For this review, take the finished solid that the model builds, in its own axes (mm). Face numbers are marked on the shaded views. A direction names the side the tool comes from. Coordinates: 2 decimals unless noted, no trailing zeros. Write each loop counter-clockwise with the first axis right and the second up, starting at its lowest first coordinate (ties: lowest second). Pieces come first, ordered by that corner, then holes.
```python
from build123d import *

# Parameters (mm, degrees)
SKETCH_A01_8_R     = 6.85
SKETCH_A01_8_W     = 10
SKETCH_A01_8_H     = 10
EXTRUDE1_DEPTH     = 100
CUT_EXTRUDE1_DEPTH = 101
CIRPATTERN1_COUNT  = 2
CIRPATTERN1_ANGLE  = 90
CUT_EXTRUDE2_DEPTH = 101
EXTRUDE3_DEPTH     = 100


with BuildPart() as part:
    # Sketch A01-8 → Extrude1 (new body)
    with BuildSketch(Plane.XY):
        Polygon((-16.5, -11), (-16.5, -9.5), (-15.863961, -9.5), (-10.14602885, -3.78206785), (-10.14602885, 3.78206785), (-15.863961, 9.5), (-16.5, 9.5), (-16.5, 11), (-21, 11), (-21, 4), (-25, 4), (-25, 25), (25, 25), (25, 4), (21, 4), (21, 11), (16.5, 11), (16.5, 9.5), (15.863961, 9.5), (10.14602885, 3.78206785), (10.14602885, -3.78206785), (15.863961, -9.5), (16.5, -9.5), (16.5, -11), (21, -11), (21, -4), (25, -4), (25, -25), (4, -25), (4, -21), (11, -21), (11, -16.5), (9.5, -16.5), (9.5, -15.863961), (3.78206785, -10.14602885), (-3.78206785, -10.14602885), (-9.5, -15.863961), (-9.5, -16.5), (-11, -16.5), (-11, -21), (-4, -21), (-4, -25), (-25, -25), (-25, -4), (-21, -4), (-21, -11), align=None)
        Circle(SKETCH_A01_8_R, mode=Mode.SUBTRACT)
        with Locations((-18, -18)):
            Rectangle(SKETCH_A01_8_W, SKETCH_A01_8_H, mode=Mode.SUBTRACT)
        with Locations((18, -18)):
            Rectangle(SKETCH_A01_8_W, SKETCH_A01_8_H, mode=Mode.SUBTRACT)
        Polygon((23, 13), (16.535534, 13), (14.035536811, 10.500002811), (-14.035536811, 10.500002811), (-16.535534, 13), (-23, 13), (-23, 23), (23, 23), align=None, mode=Mode.SUBTRACT)
    extrude(amount=-EXTRUDE1_DEPTH)

    # Sketch1 → Cut-Extrude1 (cut, through all)
    with BuildSketch(Plane.XY):
        Polygon((-16.5, -13), (-9.340048075, -5.840048075), (-5.840048075, -9.340048075), (-13, -16.5), align=None)
    cut_extrude1 = extrude(amount=-CUT_EXTRUDE1_DEPTH, mode=Mode.SUBTRACT)

    # CirPattern1: Cut-Extrude1 ×2 about axis
    cirpattern1_axis = Axis((0, 0, 0), (0, 0, 1))
    for i in range(1, CIRPATTERN1_COUNT):
        add(cut_extrude1.rotate(cirpattern1_axis, i * CIRPATTERN1_ANGLE / (CIRPATTERN1_COUNT - 1)), mode=Mode.SUBTRACT)

    # Sketch2 → Cut-Extrude2 (cut, through all)
    with BuildSketch(Plane.XY):
        with BuildLine():
            Line((-14.035536811, 10.500002811), (-10.114441476, 6.578907476))
            ThreePointArc((-10.114441476, 6.578907476), (0, 10.768446311), (10.114441476, 6.578907476))
            Line((10.114441476, 6.578907476), (14.035536811, 10.500002811))
            ThreePointArc((14.035536811, 10.500002811), (0, 16.313712513), (-14.035536811, 10.500002811))
        make_face()
    extrude(amount=-CUT_EXTRUDE2_DEPTH, mode=Mode.SUBTRACT)

    # Sketch3 → Extrude3 (add, through all)
    with BuildSketch(Plane.XY):
        Polygon((-11, 23), (-11, 15), (-7, 15), (-7, 17), (-9.5, 17), (-9.5, 23), align=None)
        Polygon((11, 23), (11, 15), (7, 15), (7, 17), (9.5, 17), (9.5, 23), align=None)
    extrude(amount=-EXTRUDE3_DEPTH)


solid = part.part
```
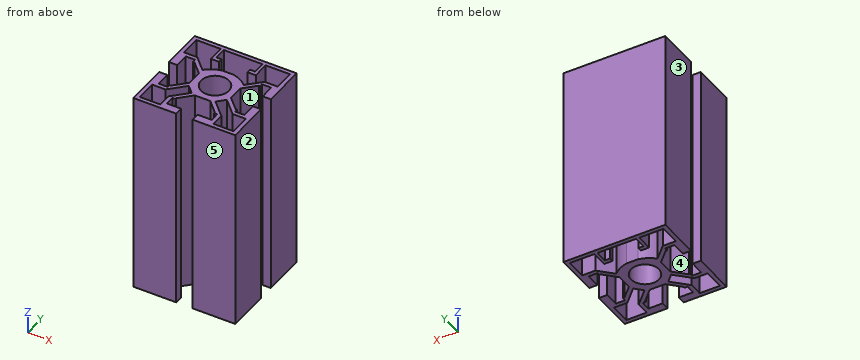
Q1. Add section A-A (y = 0). State the section outline as (x, z) points.
Ans:
outline: (-10.15, -100) - (-6.85, -100) - (-6.85, 0) - (-10.15, 0) - close; (6.85, -100) - (10.15, -100) - (10.15, 0) - (6.85, 0) - close
Q2. Add section C-C (x = 0). State the section outline as (y, z) points, then the cut area to 3 significant figures.
Ans:
outline: (-10.15, -100) - (-6.85, -100) - (-6.85, 0) - (-10.15, 0) - close; (6.85, -100) - (10.5, -100) - (10.5, 0) - (6.85, 0) - close; (23, -100) - (25, -100) - (25, 0) - (23, 0) - close
area: 895 mm2
Q3. Draft analysis for pull direction X (two halves, no side actions). For the marked faces 1, 2 and 3, state which applies: +X half, -X half, draft (parallel to the pull), parting line (faces both ways), or undercut.
Ans:
face 1: undercut
face 2: +X half
face 3: -X half
Q4. Tool access review of the marked faces 4 and 5: name each direction out of +Z, -Z, +X, -X, +Y, -Y from which nothing blocks a thin tool from reaching the whole face with its end or side.
Ans:
face 4: +Z, -Z
face 5: +Z, -Z, +X, -X, -Y
Q5. For probe 1 along Y at (x, z) = (0.5, -22); probe 2 along Y at (x, z) = (19.5, -74.5); probe 3 along Y at (x, z) = (2.5, -76), list the stretches that pass through material, from the lowest coordinate up.
Ans:
probe 1: y = -10.15 to -6.83, 6.83 to 10.5, 23 to 25
probe 2: y = -25 to -23, -13 to -11, 11 to 13, 23 to 25
probe 3: y = -10.15 to -6.38, 6.38 to 10.5, 23 to 25
Q6. Clearance check with a flat-ended pin moving along its axis: pin 1 Ø2 at (y, z) = (2.5, -25.5) entering from +X. State where the tip first meets the part, or that it passes through.
Ans:
pin 1: stops at x = 10.15
Q7. Add section B-B (x = 18). State the section outline as (y, z) points, then the cut area to 3 significant figures.
Ans:
outline: (-25, -100) - (-23, -100) - (-23, 0) - (-25, 0) - close; (-13, -100) - (-11, -100) - (-11, 0) - (-13, 0) - close; (11, -100) - (13, -100) - (13, 0) - (11, 0) - close; (23, -100) - (25, -100) - (25, 0) - (23, 0) - close
area: 800 mm2
Q8. Add section D-D (y = -8). State the section outline as (x, z) points, then the cut area to 3 significant figures.
Ans:
outline: (-25, -100) - (-21, -100) - (-21, 0) - (-25, 0) - close; (-14.36, -100) - (-11.5, -100) - (-11.5, 0) - (-14.36, 0) - close; (-7.18, -100) - (7.18, -100) - (7.18, 0) - (-7.18, 0) - close; (11.5, -100) - (14.36, -100) - (14.36, 0) - (11.5, 0) - close; (21, -100) - (25, -100) - (25, 0) - (21, 0) - close
area: 2,810 mm2
